The listing builds one solid part. Answer for the finished solid, in the listing's coordinates (mm). A direction names the side the tool comes from. Coordinates: 2 decimals unless noted, no trailing zeros. Write each loop counter-clockwise with the first axis right and the second up, starting at its lowest first coordinate (ties: lowest second). Pieces come first, ordered by that corner, then holes. Notation, with made-up numbers: M 50.25,-10.5 L 102.25,-10.5 A30 ccw 102.25,25.5 Z; hole C 25.5,83.25 d1. An arc over 180 degrees is marked long. Answer as a JSON object with one key per item and string values. Group by question number.
from build123d import *

# Parameters (mm, degrees)
F1_DEPTH       = 10
F3_D           = 3.3
F3_CSINK_D     = 6.72
F3_CSINK_ANGLE = 90
F5_D           = 3.3
F5_CSINK_D     = 6.72
F5_CSINK_ANGLE = 90
F6_R           = 2


with BuildPart() as f1:
    # F0 (on Top) → F1 (new body)
    with BuildSketch(Plane.XY):
        with BuildLine():
            Line((0, 15), (0, 0))
            Line((0, 0), (15, 0))
            Line((15, 0), (15, 3))
            Line((15, 3), (6, 3))
            ThreePointArc((6, 3), (3.8786796564, 3.8786796564), (3, 6))
            Line((3, 6), (3, 15))
            Line((3, 15), (0, 15))
        make_face()
    extrude(amount=F1_DEPTH)

    # F3 (through all)
    with Locations(Plane.YZ.offset(3)):
        with Locations((10, 5)):
            CounterSinkHole(F3_D / 2, F3_CSINK_D / 2, counter_sink_angle=F3_CSINK_ANGLE)

    # F5 (through all)
    with Locations(Plane(origin=(0, 3, 0), x_dir=(-1, 0, 0), z_dir=(0, 1, 0))):
        with Locations((-10, 5)):
            CounterSinkHole(F5_D / 2, F5_CSINK_D / 2, counter_sink_angle=F5_CSINK_ANGLE)

    # F6
    f6_edges = [f1.edges().sort_by_distance(p)[0] for p in [
        (0, 0, 5),
    ]]
    fillet(f6_edges, radius=F6_R)


solid = f1.part
Item 1: Consider L1, parallel to Z at x = 10, y = 0.7; L2, parallel to X at y = 6, z = 3.25; L3, parallel to Y at x = 2.75, z = 3.5. Determine where each line is inside the solid, lowest interval first. Write a range as from..to.
Item 2: A cutting plane is placed at A-A, the plane x = 10. Write down the section's boundary in (y, z), and give its area (3 significant figures).
Item 3: A tool of negligible diameter and unlimited length cuts with its end or side. For faces 1 (the face through (2, 15, 5)), 2 (the face through (3, 13.4, 3.8)), from which of +Z, -Z, +X, -X, +Y, -Y can it reach the whole face along a straight path? Write none if from no direction.
Item 4: For a pull along Y with two mould halves and no side action, classify faces 3 (the face through (0.636, 9.239, 3.536)), 4 (the face through (4, 3, 0)), 5 (the face through (3.9, 3.86, 4.93)), 6 (the face through (0.57, 0.6, 5.07)) as +Y half, -Y half, draft (parallel to the pull), parting line (faces both ways), or undercut.
Item 5: A cutting plane is placed at C-C, the plane z = 5. Write down the section's boundary in (x, y).
Item 6: Flat-ended cylindrical pins translate along their axes: pin 1 Ø6 at (y, z) = (7.5, 7.5) entering from +X; pin 2 Ø1.5 at (x, y) = (5.5, 10) entering from +Z; pin 3 Ø4 at (y, z) = (13.5, 6.5) entering from +X; pin 4 Ø4 at (x, z) = (10, 5) entering from +Y. Find the tip coordinate at first contact, or state that the pin passes through.
Item 7: A cutting plane is placed at D-D, the plane z = 1. Write down the section's boundary in (x, y), and give its area (3 significant figures).
Answer:
{
 "1": {"L1": "0..3.35, 6.65..10", "L2": "0..3", "L3": "0..7.28, 12.72..15"},
 "2": {"outline": "M 0,0 L 3,0 L 3,1.64 L 1.29,3.35 L 0,3.35 Z; M 0,6.65 L 1.29,6.65 L 3,8.36 L 3,10 L 0,10 Z", "area": "17.2 mm2"},
 "3": {"face 1": "+Z, -Z, +X, -X, +Y", "face 2": "+Z, -Z, +X, +Y"},
 "4": {"face 3": "undercut", "face 4": "draft", "face 5": "+Y half", "face 6": "-Y half"},
 "5": {"outline": "M 0,2 A2 ccw 2,0 L 8.35,0 L 8.35,1.29 L 6.64,3 L 6,3 A3 cw 3,6 L 3,6.64 L 1.29,8.35 L 0,8.35 Z; M 0,11.65 L 1.29,11.65 L 3,13.36 L 3,15 L 0,15 Z; M 11.65,0 L 15,0 L 15,3 L 13.36,3 L 11.65,1.29 Z"},
 "6": {"pin 1": "x = 3.4", "pin 2": "through", "pin 3": "x = 3", "pin 4": "y = 1.64"},
 "7": {"outline": "M 0,2 A2 ccw 2,0 L 15,0 L 15,3 L 6,3 A3 cw 3,6 L 3,15 L 0,15 Z", "area": "82.1 mm2"}
}
